```python
from build123d import *

# Parameters (mm, degrees)
SKETCH1_W                       = 31
SKETCH1_H                       = 56
BOSS_EXTRUDE1_DEPTH             = 6.35
SKETCH2_R                       = 11.1125
BOSS_EXTRUDE2_DEPTH             = 24.15253802
SKETCH3_R                       = 7.54126
CUT_EXTRUDE1_DEPTH              = 31.50253802
SKETCH4_W                       = 26
SKETCH4_H                       = 44
CUT_EXTRUDE2_DEPTH              = 1.27
FILLET1_R                       = 3.175
FILLET1_OF_MIRROR2_R            = 3.175
F_10_24_TAPPED_HOLE1_AT_2_COUNT = 2
F_10_24_TAPPED_HOLE1_AT_2_PITCH = 28


with BuildPart() as part:
    # Sketch1 → Boss-Extrude1 (new body)
    with BuildSketch(Plane(origin=(0, 0, 0), x_dir=(0, 0, -1), z_dir=(1, 0, 0))):
        with Locations((-3.5, 28)):
            Rectangle(SKETCH1_W, SKETCH1_H)
    boss_extrude1 = extrude(amount=BOSS_EXTRUDE1_DEPTH)

    # Mirror1: Boss-Extrude1 across plane
    add(boss_extrude1.mirror(Plane.ZX))

    # Sketch2 → Boss-Extrude2 (add)
    with BuildSketch(Plane(origin=(6.35, 0, 0), x_dir=(0, 0, -1), z_dir=(1, 0, 0))):
        Circle(SKETCH2_R)
    extrude(amount=BOSS_EXTRUDE2_DEPTH)

    # Sketch3 → Cut-Extrude1 (cut, through all)
    with BuildSketch(Plane.ZY):
        Circle(SKETCH3_R)
    extrude(amount=-CUT_EXTRUDE1_DEPTH, mode=Mode.SUBTRACT)

    # Sketch4 → Cut-Extrude2 (cut)
    with BuildSketch(Plane.ZY):
        with Locations((6, 34)):
            Rectangle(SKETCH4_W, SKETCH4_H)
    cut_extrude2 = extrude(amount=-CUT_EXTRUDE2_DEPTH, mode=Mode.SUBTRACT)

    # Fillet1
    fillet1_edges = [part.edges().sort_by_distance(p)[0] for p in [
        (0.635, 12, -7),
    ]]
    fillet(fillet1_edges, radius=FILLET1_R)

    # Mirror2: Cut-Extrude2 across plane
    add(cut_extrude2.mirror(Plane.ZX), mode=Mode.SUBTRACT)

    # Fillet1 of Mirror2
    fillet1_of_mirror2_edges = [part.edges().sort_by_distance(p)[0] for p in [
        (0.635, -12, -7),
    ]]
    fillet(fillet1_of_mirror2_edges, radius=FILLET1_OF_MIRROR2_R)

    # Sketch5 → #10-24 Tapped Hole1 (revolve, cut)
    with BuildSketch(Plane(origin=(1.27, 50, 5), x_dir=(0, 0, 1), z_dir=(0, 1, 0))):
        Polygon((0, 0), (0, 16.090824014), (1.89865, 14.95), (1.89865, 0), align=None)
    f_10_24_tapped_hole1 = revolve(axis=Axis((-5.08, 50, 5), (1, 0, 0)), mode=Mode.SUBTRACT)

    # #10-24 Tapped Hole1 at 2: #10-24 Tapped Hole1 ×2
    with Locations(*[(0, -i * F_10_24_TAPPED_HOLE1_AT_2_PITCH, 0) for i in range(1, F_10_24_TAPPED_HOLE1_AT_2_COUNT)]):
        add(f_10_24_tapped_hole1, mode=Mode.SUBTRACT)

    # Mirror3: #10-24 Tapped Hole1 across plane
    add(f_10_24_tapped_hole1.mirror(Plane.ZX), mode=Mode.SUBTRACT)

    # Mirror3 copy 1 sketch → Mirror3 copy 1 (revolve, cut)
    with BuildSketch(Plane(origin=(1.27, -22, 5), x_dir=(0, 0, 1), z_dir=(0, -1, 0))):
        Polygon((0, 0), (0, -16.090824014), (1.89865, -14.95), (1.89865, 0), align=None)
    revolve(axis=Axis((-5.08, -22, 5), (-1, 0, 0)), mode=Mode.SUBTRACT)


solid = part.part
```
Could you check a few things on this model? Use its own coordinates, in mm. A direction names the side the tool comes from. Give positions to 0.01 mm unless a question says otherwise; leave off trailing zeros. Order: outer loops, then holes, each group sorted by start corner. A loop starts at its lowest first (then second) coordinate and runs counter-clockwise, first axis right, second up.
Q1. I'm going to push flat-ended pins straight in: P1, Ø5, axis at y = -50, z = 5, coming from the +X side; P2, Ø8, axis at y = 24, z = 12, coming from the -X side; P3, Ø1, axis at x = 0.5, z = 6.5, coming from the -Y side. Where does each tip first touch, or does it pass through?
Q2. Suppose I cut it at B-B, the plane z = 14. Write out the boundary of the cut face in (x, y), and give its area (3 significant figures).
Q3. For faces 1 (the cylindrical face through (0.64, -12.91, -6.05)), 2 (the flat face through (1.27, 34, 6)), 3 (the cylindrical face through (18.26, 3.34, -10.6)), which set-ups out of +Z, -Z, +X, -X, +Y, -Y let a thin tool reach every point of the face, with its end or its side?
Q4. Suppose I cut it at C-C, the plane x = 15.5. Write out the boundary of the cut face in (y, z) (1 decimal), and give its area (3 significant figures).
Q5. Suppose I cut it at D-D, the plane y = 14. Write out the boundary of the cut face in (x, z), and give its area (3 significant figures).
Q6. We'd pull the mould along Y, two halves only. Please class faces 4 (the cylindrical face through (0.64, 12.91, -6.05)), 5 (the flat face through (3, 1, -12)), 6 (the cylindrical face through (3.77, -48.4, 6.02)), 7 (the cylindrical face through (15.038, 7.477, -0.982)): +Y half, -Y half, draft (parallel to the pull), parting line (faces both ways), or undercut.
Q7. If I drill on line 1 along Y through (x, z) = (19.5, 0); line 2 along Y through (x, z) = (2, 5); line 3 along Z through (x, y) = (2, 22), over which ranges is the centre line in solid material (lowest first)?
Q8. Suppose I cut it at A-A, the plane y = -50. Write out the boundary of the cut face in (x, z).
Solution:
1. P1: stops at x = 6.35
1. P2: stops at x = 1.27
1. P3: stops at y = -12
2. outline: (0, -12) - (1.27, -12) - (1.27, -56) - (6.35, -56) - (6.35, 56) - (1.27, 56) - (1.27, 12) - (0, 12) - close
2. area: 599 mm2
3. face 1: +Z, -X, -Y
3. face 2: +Z, -X, +Y
3. face 3: +X
4. outline: circle Ø22.2 at (0, 0); hole circle Ø15.1 at (0, 0)
4. area: 209 mm2
5. outline: (0, -12) - (6.35, -12) - (6.35, 19) - (1.27, 19) - (1.27, -6.77) - (0, -6.77) - close
5. area: 164 mm2
6. face 4: +Y half
6. face 5: draft
6. face 6: undercut
6. face 7: undercut
7. line 1: y = -11.11 to -7.54, 7.54 to 11.11
7. line 2: y = -56 to -51.9, -48.1 to -23.9, -20.1 to -5.65, 5.65 to 20.1, 23.9 to 48.1, 51.9 to 56
7. line 3: z = -12 to 3.1, 6.9 to 19
8. outline: (0, -12) - (6.35, -12) - (6.35, 3.1) - (1.27, 3.1) - (1.27, -7) - (0, -7) - close; (1.27, 6.9) - (6.35, 6.9) - (6.35, 19) - (1.27, 19) - close
